Here's the drawing with two shaded views (mm, measured from the low corner). I have some questions. Coordinates: 2 decimals unless noted, no trailing zeros. Order: outer loops, then holes, each group sorted by start corner. A loop starts at its lowest first (then second) coordinate and runs counter-clockwise, first axis right, second up. Notation, with made-up numbers: (73.5, -8.75) -> (90.5, -8.75) arc R17 ccw to (90.5, 16.25) -> close; hole circle Ø7 at (13.5, 89). An arc over 180 degrees is marked (long way). Answer in a Markdown table with one row per item. Add a question column.
1. Imagine slicing it at C-C on y = 31. Write out the boundary of the cut face in (x, z).
2. If I drill on line 1 along Y through (x, z) = (36.25, 13); line 2 along Y through (x, z) = (21, 24.2); line 3 along Z through (x, y) = (21, 29), over which ranges is the centre line in solid material (lowest first)? Write a range as [from, to].
3. Imagine slicing it at D-D on z = 23.75. Write out the boundary of the cut face in (x, y), plus the area to 3 significant figures.
4. Imagine slicing it at A-A on z = 13. Write out the boundary of the cut face in (x, y).
5. We'd pull the mould along Z, two halves only. Please class the marked faces 1, 2 and 3: pulls with the +Z half, pulls with the -Z half, needs draft (parallel to the pull), parting line crosses it, or undercut.
6. Will these pins go through, and if not, where does the flat tip stop? pin 1 (0.9 mm diameter, centred on x = 20.5, y = 18.5, fed in from +Z); pin 2 (5.5 mm diameter, centred on x = 5.75, y = 5, fed in from +Z); pin 3 (8 mm diameter, centred on x = 22.5, z = 12.5, fed in from -Y).
7. Imagine slicing it at B-B on x = 5.75. Write out the boundary of the cut face in (y, z).
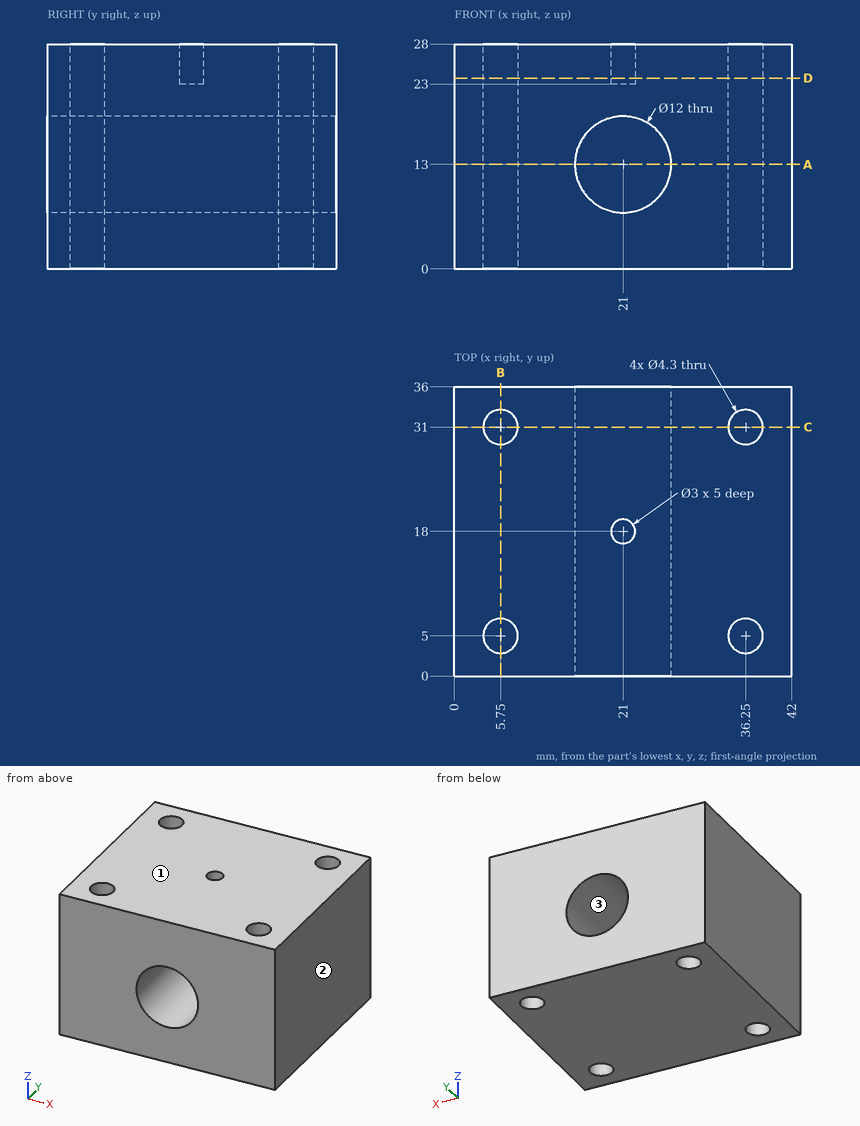
Answers follow:
| question | item | result |
|---|---|---|
| 1 | outline | (0, 0) -> (3.6, 0) -> (3.6, 28) -> (0, 28) -> close; (7.9, 0) -> (34.1, 0) -> (34.1, 28) -> (7.9, 28) -> close; (38.4, 0) -> (42, 0) -> (42, 28) -> (38.4, 28) -> close; hole circle Ø12 at (21, 13) |
| 2 | line 1 | y = [0, 2.85], [7.15, 28.85], [33.15, 36] |
| 2 | line 2 | y = [0, 16.5], [19.5, 36] |
| 2 | line 3 | z = [0, 7], [19, 28] |
| 3 | outline | (0, 0) -> (42, 0) -> (42, 36) -> (0, 36) -> close; hole circle Ø4.3 at (5.75, 5); hole circle Ø4.3 at (5.75, 31); hole circle Ø3 at (21, 18); hole circle Ø4.3 at (36.25, 5); hole circle Ø4.3 at (36.25, 31) |
| 3 | area | 1,450 mm² |
| 4 | outline | (0, 0) -> (15, 0) -> (15, 36) -> (0, 36) -> close; (27, 0) -> (42, 0) -> (42, 36) -> (27, 36) -> close; hole circle Ø4.3 at (5.75, 5); hole circle Ø4.3 at (5.75, 31); hole circle Ø4.3 at (36.25, 5); hole circle Ø4.3 at (36.25, 31) |
| 5 | face 1 | pulls with the +Z half |
| 5 | face 2 | needs draft |
| 5 | face 3 | undercut |
| 6 | pin 1 | stops at z = 23 |
| 6 | pin 2 | stops at z = 28 |
| 6 | pin 3 | passes through |
| 7 | outline | (0, 0) -> (2.85, 0) -> (2.85, 28) -> (0, 28) -> close; (7.15, 0) -> (28.85, 0) -> (28.85, 28) -> (7.15, 28) -> close; (33.15, 0) -> (36, 0) -> (36, 28) -> (33.15, 28) -> close |
